from build123d import *

# Parameters (mm, degrees)
BOSS_EXTRUDE1_DEPTH = 10
CUT_EXTRUDE1_DEPTH  = 8
CUT_EXTRUDE2_DEPTH  = 8
SKETCH4_R           = 2.5
CUT_EXTRUDE3_DEPTH  = 8
BOSS_EXTRUDE2_DEPTH = 0.5


with BuildPart() as part:
    # Sketch1 → Boss-Extrude1 (new body)
    with BuildSketch(Plane(origin=(0, 0, 0), x_dir=(1, 0, 0), z_dir=(0, 1, 0))):
        with BuildLine():
            Line((-74.5, 40), (74.5, 40))
            ThreePointArc((74.5, 40), (80.156854249, 37.656854249), (82.5, 32))
            Line((82.5, 32), (82.5, -32))
            ThreePointArc((82.5, -32), (80.156854249, -37.656854249), (74.5, -40))
            Line((74.5, -40), (-74.5, -40))
            ThreePointArc((-74.5, -40), (-80.156854249, -37.656854249), (-82.5, -32))
            Line((-82.5, -32), (-82.5, 32))
            ThreePointArc((-82.5, 32), (-80.156854249, 37.656854249), (-74.5, 40))
        make_face()
    extrude(amount=BOSS_EXTRUDE1_DEPTH)

    # Sketch2 → Cut-Extrude1 (cut)
    with BuildSketch(Plane(origin=(0, 10, 0), x_dir=(1, 0, 0), z_dir=(0, 1, 0))):
        with BuildLine():
            Line((-76.5, 38), (76.5, 38))
            ThreePointArc((76.5, 38), (79.328427125, 36.828427125), (80.5, 34))
            Line((80.5, 34), (80.5, -34))
            ThreePointArc((80.5, -34), (79.328427125, -36.828427125), (76.5, -38))
            Line((76.5, -38), (-76.5, -38))
            ThreePointArc((-76.5, -38), (-79.328427125, -36.828427125), (-80.5, -34))
            Line((-80.5, -34), (-80.5, 34))
            ThreePointArc((-80.5, 34), (-79.328427125, 36.828427125), (-76.5, 38))
        make_face()
    extrude(amount=-CUT_EXTRUDE1_DEPTH, mode=Mode.SUBTRACT)

    # Sketch3 → Cut-Extrude2 (cut)
    with BuildSketch(Plane(origin=(0, 2, 0), x_dir=(1, 0, 0), z_dir=(0, 1, 0))):
        with BuildLine():
            Line((-71.5, -8), (-44.5, -8))
            ThreePointArc((-44.5, -8), (-41.671572875, -9.171572875), (-40.5, -12))
            Line((-40.5, -12), (-40.5, -29))
            ThreePointArc((-40.5, -29), (-41.671572875, -31.828427125), (-44.5, -33))
            Line((-44.5, -33), (-71.5, -33))
            ThreePointArc((-71.5, -33), (-74.328427125, -31.828427125), (-75.5, -29))
            Line((-75.5, -29), (-75.5, -12))
            ThreePointArc((-75.5, -12), (-74.328427125, -9.171572875), (-71.5, -8))
        make_face()
        with BuildLine():
            Line((-44.5, 9.198469839), (-36.645114423, 9.198469839))
            ThreePointArc((-36.645114423, 9.198469839), (-29.446644584, 2), (-36.645114423, -5.198469839))
            Line((-36.645114423, -5.198469839), (-44.5, -5.198469839))
            ThreePointArc((-44.5, -5.198469839), (-51.698469839, 2), (-44.5, 9.198469839))
        make_face()
    extrude(amount=-CUT_EXTRUDE2_DEPTH, mode=Mode.SUBTRACT)

    # Sketch4 → Cut-Extrude3 (cut)
    with BuildSketch(Plane(origin=(82.5, 0, 0), x_dir=(0, 0, -1), z_dir=(1, 0, 0))):
        with Locations((-20, 4.917165975)):
            Circle(SKETCH4_R)
        with BuildLine():
            Line((-4, 8), (4, 8))
            ThreePointArc((4, 8), (7, 5), (4, 2))
            Line((4, 2), (-4, 2))
            ThreePointArc((-4, 2), (-7, 5), (-4, 8))
        make_face()
        with BuildLine():
            Line((15, 7.5), (25, 7.5))
            ThreePointArc((25, 7.5), (27.5, 5), (25, 2.5))
            Line((25, 2.5), (15, 2.5))
            ThreePointArc((15, 2.5), (12.5, 5), (15, 7.5))
        make_face()
    extrude(amount=-CUT_EXTRUDE3_DEPTH, mode=Mode.SUBTRACT)

    # Sketch6 → Boss-Extrude2 (add)
    with BuildSketch(Plane(origin=(0, 10, 0), x_dir=(1, 0, 0), z_dir=(0, 1, 0))):
        with BuildLine():
            Line((80.5, -34), (80.5, 34))
            ThreePointArc((80.5, 34), (79.328427125, 36.828427125), (76.5, 38))
            Line((76.5, 38), (-76.5, 38))
            ThreePointArc((-76.5, 38), (-79.328427125, 36.828427125), (-80.5, 34))
            Line((-80.5, 34), (-80.5, -34))
            ThreePointArc((-80.5, -34), (-79.328427125, -36.828427125), (-76.5, -38))
            Line((-76.5, -38), (76.5, -38))
            ThreePointArc((76.5, -38), (79.328427125, -36.828427125), (80.5, -34))
        make_face()
        with BuildLine():
            Line((-76, 37.5), (76, 37.5))
            ThreePointArc((76, 37.5), (78.828427125, 36.328427125), (80, 33.5))
            Line((80, 33.5), (80, -33.5))
            ThreePointArc((80, -33.5), (78.828427125, -36.328427125), (76, -37.5))
            Line((76, -37.5), (-76, -37.5))
            ThreePointArc((-76, -37.5), (-78.828427125, -36.328427125), (-80, -33.5))
            Line((-80, -33.5), (-80, 33.5))
            ThreePointArc((-80, 33.5), (-78.828427125, 36.328427125), (-76, 37.5))
        make_face(mode=Mode.SUBTRACT)
    extrude(amount=-BOSS_EXTRUDE2_DEPTH)


solid = part.part
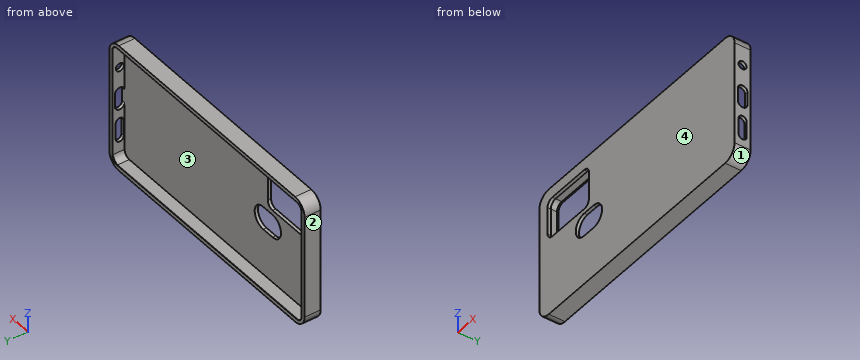
Read the model definition and answer for the solid it produces. Units are mm, in the model's axes. Face numbers are marked on the shaded views. Round coordinates to 2 decimals unless told otherwise and drop trailing zeros. Write each loop counter-clockwise with the first axis right and the second up, starting at its lowest first coordinate (ties: lowest second). Pieces come first, ordered by that corner, then holes. Notation, with made-up numbers: M 83.25,-7 L 130.25,-7 A20 cw 130.25,3 Z; hole C 37.5,-39 d2. An arc over 180 degrees is marked long. Use a Markdown table: item, result.
1) The part is cut by section D-D (z = -5.5). Write down the section's boundary in (x, y).
Answers follow:
| item | result |
|---|---|
| outline | M -82.5,0 L -50.79,0 L -50.79,2 L -80.5,2 L -80.5,9.5 L -80,9.5 L -80,10 L -82.5,10 Z; M -30.35,0 L 82.5,0 L 82.5,2.4 L 80.5,2.4 L 80.5,2 L -30.35,2 Z; M 80,9.5 L 80.5,9.5 L 80.5,7.6 L 82.5,7.6 L 82.5,10 L 80,10 Z |
2) The part is cut by section C-C (x = 62.5). Write down the section's boundary in (y, z).
Answers follow:
| item | result |
|---|---|
| outline | M 0,-40 L 10,-40 L 10,-37.5 L 9.5,-37.5 L 9.5,-38 L 2,-38 L 2,38 L 9.5,38 L 9.5,37.5 L 10,37.5 L 10,40 L 0,40 Z |
3) The part is cut by section B-B (x = -55). Write down the section's boundary in (y, z).
Answers follow:
| item | result |
|---|---|
| outline | M 0,-40 L 10,-40 L 10,-37.5 L 9.5,-37.5 L 9.5,-38 L 2,-38 L 2,8 L 0,8 Z; M 0,33 L 2,33 L 2,38 L 9.5,38 L 9.5,37.5 L 10,37.5 L 10,40 L 0,40 Z |
4) The part is cut by section A-A (z = 20). Write down the section's boundary in (x, y), plus the area to 4 significant figures.
Answers follow:
| item | result |
|---|---|
| outline | M -82.5,0 L -75.5,0 L -75.5,2 L -80.5,2 L -80.5,9.5 L -80,9.5 L -80,10 L -82.5,10 Z; M -40.5,0 L 82.5,0 L 82.5,2.42 L 80.5,2.42 L 80.5,2 L -40.5,2 Z; M 80,9.5 L 80.5,9.5 L 80.5,7.42 L 82.5,7.42 L 82.5,10 L 80,10 Z |
| area | 282.5 mm2 |
5) Flat-ended cylindrical pins translate along their axes: pin 1 (1.5 mm diameter, centred on x = 8, z = 7.5, fed in from -Y); pin 2 (23 mm diameter, centred on x = -17, z = -4, fed in from +Y). Find the tip coordinate at first contact, or state that the pin passes through.
Answers follow:
| item | result |
|---|---|
| pin 1 | stops at y = 0 |
| pin 2 | stops at y = 2 |
6) Straight lines are drawn through the part: line 1 along Z through (x, y) = (48, 2.75); line 2 along X through (y, z) = (8, -16); line 3 along Y through (x, z) = (82, 20). For each, find the intervals that lie inside material, in ascending order. Write a range as [from, to].
Answers follow:
| item | result |
|---|---|
| line 1 | z = [-40, -38], [38, 40] |
| line 2 | x = [-82.5, -80.5], [80.5, 82.5] |
| line 3 | y = [0, 2.42], [7.42, 10] |
7) For a pull along X with two mould halves and no side action, classify the marked faces 1, 2, 3 and 4 as pulls with the +X half, pulls with the -X half, needs draft (parallel to the pull), parting line crosses it, or undercut.
Answers follow:
| item | result |
|---|---|
| face 1 | pulls with the +X half |
| face 2 | pulls with the -X half |
| face 3 | undercut |
| face 4 | needs draft |
